Design review of the part built by this model. Coordinates are the model's own, in mm. A direction names the side the tool comes from. Give positions to 0.01 mm unless a question says otherwise; leave off trailing zeros. Loops run counter-clockwise (first coordinate to the right, second up) from the corner with the lowest first, then second, coordinate; pieces in that order, holes last. Notation, with made-up numbers: (-7.5, -9.5) -> (44.5, -9.5) arc R26 cw to (44.5, 12.5) -> close; hole circle Ø2 at (20.25, 79.5). An arc over 180 degrees is marked (long way). Answer in a Markdown table with one row per item. Add a question column.
(1) Consider section C-C on y = 0.55. Write out the cut boundary in (x, z).
(2) For faces 1 (the flat face through (19, 4, 0)), 2 (the cylindrical face through (13.1, 2.46, 19.43)), 3 (the cylindrical face through (-14.84, 2.46, 13.76)), list the 3-axis set-ups (+Z, -Z, +X, -X, +Y, -Y) from which the entire face can be reached by the end or side of a thin tool; tool diameter is ignored.
(3) Consider section D-D on z = -11. Write out the cut boundary in (x, y), then the cut area to 3 significant figures.
(4) Consider section B-B on z = 15. Write out the cut boundary in (x, y).
(5) For line 1 (Z direction, x = 15, y = 3.3); line 2 (Z direction, x = -15, y = 1.9); line 3 (X direction, y = 3.7, z = -10.5), list the stretches that pass through material, from the lowest coordinate up.
(6) Draft analysis for pull direction X (two halves, no side actions). For faces 4 (the flat face through (20, 2, 0)), 5 (the cylindrical face through (-14.079, 2.465, -15.845)), 6 (the flat face through (1.6, 5, -19.2)), 7 (the flat face through (0, 2, -2)), state which applies: +X half, -X half, draft (parallel to the pull), parting line (faces both ways), or undercut.
(7) For pin 1 (10.5 mm diameter, centred on x = -5.5, z = 0.5, fed in from +Y); pin 2 (2.5 mm diameter, centred on x = 0.5, y = 4, fed in from +Z); pin 3 (1 mm diameter, centred on x = 0, y = 1, fed in from +Z), all flat-tipped, find the tip position at first contact; note any pin that passes through.
(8) Consider section A-A on x = 15. Write out the cut boundary in (y, z).
Autodesk Inventor part; units mm, degrees
ref_plane "YZ Plane" through (0, 0, 0) normal (1, 0, 0) x (0, 1, 0)
ref_plane "XZ Plane" through (0, 0, 0) normal (0, 1, 0) x (-1, 0, 0)
ref_plane "XY Plane" through (0, 0, 0) normal (0, 0, 1) x (1, 0, 0)
sketch "Sketch1" plane through (0, 0, 0) normal (0, 1, 0) x (-1, 0, 0)
  line L0 (19, 19) -> (-19, 19) construction
  line L1 (-19, 19) -> (-19, -19) construction
  line L2 (-19, -19) -> (19, -19) construction
  line L3 (19, -19) -> (19, 19) construction
  line L4 (19, 19) -> (-19, -19) construction
  line L5 (-19, 19) -> (19, -19) construction
  circle A0 centre (15, -15) radius 1.25
  circle A1 centre (-15, -15) radius 1.25
  circle A2 centre (15, 15) radius 1.25
  circle A3 centre (-15, 15) radius 1.25
  line L6 (20, 20) -> (-20, 20)
  line L7 (-20, 20) -> (-20, -20)
  line L8 (-20, -20) -> (20, -20)
  line L9 (20, -20) -> (20, 20)
  line L10 (20, 20) -> (-20, -20) construction
  line L11 (-20, 20) -> (20, -20) construction
  point P0 (0, 0)
  dimension "d0" = 38
  dimension "d1" = 38
  dimension "d2" = 2.5
  dimension "d3" = 2.5
  dimension "d4" = 2.5
  dimension "d5" = 2.5
  dimension "d6" = 4
  dimension "d7" = 4
  dimension "d8" = 4
  dimension "d9" = 4
  dimension "d10" = 40
  dimension "d11" = 40
extrude "Extrusion1" add sketch "Sketch1" along normal blind 5
sketch "Sketch2" plane through (0, 5, 0) normal (0, 1, 0) x (1, 0, 0)
  line L0 (-12.5, 19) -> (-12.5, 12.5)
  line L1 (-12.5, 12.5) -> (-19, 12.5)
  line L2 (-19, 12.5) -> (-19, -12.5)
  line L3 (-20, 20) -> (-20, -20)
  line L4 (-19, -12.5) -> (-12.5, -12.5)
  line L5 (-12.5, -12.5) -> (-12.5, -20)
  line L6 (-12.5, -20) -> (12.5, -20)
  line L7 (12.5, -20) -> (12.5, -12.5)
  line L8 (12.5, -12.5) -> (19, -12.5)
  line L9 (19, -12.5) -> (19, 12.5)
  line L10 (19, 12.5) -> (12.5, 12.5)
  line L11 (12.5, 12.5) -> (12.5, 19)
  line L12 (12.5, 19) -> (-12.5, 19)
  point P0 (0, 0)
  dimension "d14" = 25
  dimension "d15" = 6.5
  dimension "d16" = 25
  dimension "d17" = 7.5
  dimension "d18" = 6.5
  dimension "d19" = 6.5
  dimension "d20" = 25
  dimension "d21" = 6.5
  dimension "d22" = 12.5
  dimension "d24" = 12.5
extrude "Extrusion2" cut sketch "Sketch2" against normal blind 3
sketch "Sketch3" plane through (0, 2, 0) normal (0, 1, 0) x (1, 0, 0)
  line L0 (12.5, -12.5) -> (12.5, -20)
  line L1 (-12.5, -20) -> (12.5, -20)
  line L2 (12.5, -20) -> (12.5, -16)
  line L3 (12.5, -16) -> (-12.5, -16)
  line L4 (-12.5, -16) -> (-12.5, -20)
  point P0 (0, 0)
  dimension "d27" = 4
extrude "Extrusion3" cut sketch "Sketch3" against normal through all
fillet "Fillet1" radius 2 10 edges at (-20, 2.5, -20) (20, 2.5, -20) (-20, 2.5, 20) (20, 2.5, 20) (-12.5, 3.5, -12.5) (12.5, 3.5, -12.5) (12.5, 3.5, 12.5) (-12.5, 3.5, 12.5) (-12.5, 2.5, 20) (12.5, 2.5, 20)
properties part number "CameraMount2"
Values follow:
| question | item | result |
|---|---|---|
| 1 | outline | (-20, -18) arc R2 ccw to (-18, -20) -> (18, -20) arc R2 ccw to (20, -18) -> (20, 18) arc R2 ccw to (18, 20) -> (14.5, 20) arc R2 ccw to (12.5, 18) -> (12.5, 16) -> (-12.5, 16) -> (-12.5, 18) arc R2 ccw to (-14.5, 20) -> (-18, 20) arc R2 ccw to (-20, 18) -> close; hole circle Ø2.5 at (-15, -15); hole circle Ø2.5 at (-15, 15); hole circle Ø2.5 at (15, -15); hole circle Ø2.5 at (15, 15) |
| 2 | face 1 | +Y |
| 2 | face 2 | +Z, +Y, -Y |
| 2 | face 3 | +Y, -Y |
| 3 | outline | (-20, 0) -> (20, 0) -> (20, 5) -> (19, 5) -> (19, 2) -> (-19, 2) -> (-19, 5) -> (-20, 5) -> close |
| 3 | area | 86.0 mm2 |
| 4 | outline | (-20, 0) -> (-16.25, 0) -> (-16.25, 5) -> (-20, 5) -> close; (-13.75, 0) -> (13.75, 0) -> (13.75, 5) -> (12.5, 5) -> (12.5, 2) -> (-12.5, 2) -> (-12.5, 5) -> (-13.75, 5) -> close; (16.25, 0) -> (20, 0) -> (20, 5) -> (16.25, 5) -> close |
| 5 | line 1 | -20 to -16.25, -13.75 to -12.5, 12.5 to 13.75, 16.25 to 20 |
| 5 | line 2 | -20 to -16.25, -13.75 to 13.75, 16.25 to 20 |
| 5 | line 3 | -20 to -19, 19 to 20 |
| 6 | face 4 | +X half |
| 6 | face 5 | undercut |
| 6 | face 6 | draft |
| 6 | face 7 | undercut |
| 7 | pin 1 | y = 2 |
| 7 | pin 2 | z = -19 |
| 7 | pin 3 | z = 16 |
| 8 | outline | (0, -20) -> (5, -20) -> (5, -16.25) -> (0, -16.25) -> close; (0, -13.75) -> (5, -13.75) -> (5, -12.5) -> (2, -12.5) -> (2, 12.5) -> (5, 12.5) -> (5, 13.75) -> (0, 13.75) -> close; (0, 16.25) -> (5, 16.25) -> (5, 20) -> (0, 20) -> close |
